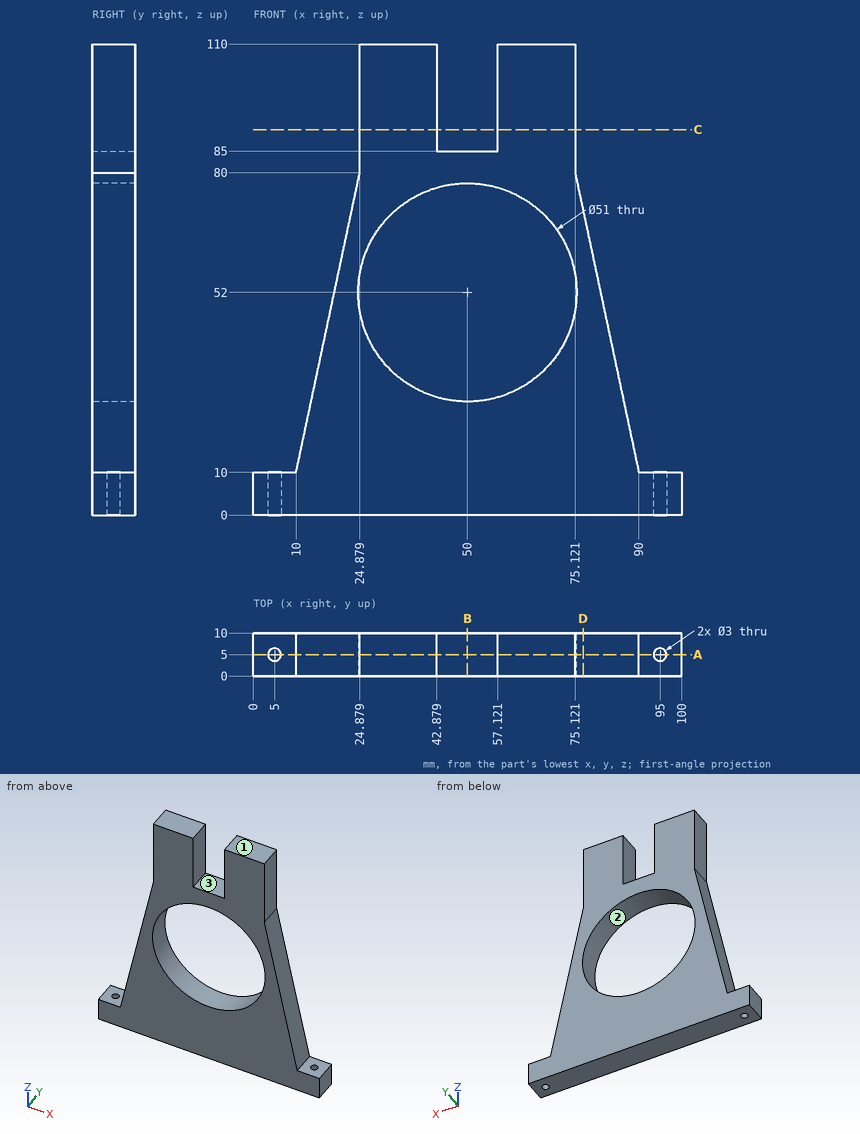
Here's the drawing with two shaded views (mm, measured from the low corner). I have some questions. Give positions to 0.01 mm unless a question says otherwise; leave off trailing zeros. Loops run counter-clockwise (first coordinate to the right, second up) from the corner with the lowest first, then second, coordinate; pieces in that order, holes last. Notation, with made-up numbers: M 81,23.25 L 106,23.25 A33 ccw 106,55.25 Z; hole C 77,-30.75 d2. An arc over 180 degrees is marked long. One line per item, written item: value.
1) Imagine slicing it at C-C on z = 90. Write out the boundary of the cut face in (x, y), and give its area (3 significant figures).
Geometry check:
outline: M 24.88,0 L 42.88,0 L 42.88,10 L 24.88,10 Z; M 57.12,0 L 75.12,0 L 75.12,10 L 57.12,10 Z
area: 360 mm²
2) Please list where these lines run through material, in increasing order: line 1 (Z direction, x = 50, y = 4); line 2 (Y direction, x = 5, z = 5); line 3 (X direction, y = 6.25, z = 6.5).
Geometry check:
line 1: z = 0 to 26.5, 77.5 to 85
line 2: y = 0 to 3.5, 6.5 to 10
line 3: x = 0 to 4.17, 5.83 to 94.17, 95.83 to 100
3) Imagine slicing it at A-A on y = 5. Write out the boundary of the cut face in (x, z), and give its area (3 significant figures).
Geometry check:
outline: M 0,0 L 3.5,0 L 3.5,10 L 0,10 Z; M 6.5,0 L 93.5,0 L 93.5,10 L 90,10 L 75.12,80 L 75.12,110 L 57.12,110 L 57.12,85 L 42.88,85 L 42.88,110 L 24.88,110 L 24.88,80 L 10,10 L 6.5,10 Z; M 96.5,0 L 100,0 L 100,10 L 96.5,10 Z; hole C 50,52 d51
area: 4,610 mm²
4) Imagine slicing it at B-B on x = 50. Write out the boundary of the cut face in (y, z).
Geometry check:
outline: M 0,0 L 10,0 L 10,26.5 L 0,26.5 Z; M 0,77.5 L 10,77.5 L 10,85 L 0,85 Z
5) Imagine slicing it at D-D on x = 77. Write out the boundary of the cut face in (y, z), and give its area (3 significant figures).
Geometry check:
outline: M 0,0 L 10,0 L 10,71.16 L 0,71.16 Z
area: 712 mm²
6) Thinking about a two-plate mould opening in X: for the marked faces 1, 2 and 3, which applies, +X half, -X half, draft (parallel to the pull), parting line (faces both ways), or undercut?
Geometry check:
face 1: draft
face 2: undercut
face 3: undercut
7) I'm going to push flat-ended pins straight in: pin 1 (1.5 mm diameter, centred on y = 2.5, z = 97, fed in from +X); pin 2 (1 mm diameter, centred on x = 52, y = 3, fed in from +Z); pin 3 (6 mm diameter, centred on x = 76.5, y = 5.5, fed in from +Z); pin 4 (1.5 mm diameter, centred on y = 4.5, z = 53, fed in from +X). Where does each tip first touch, or does it pass through?
Geometry check:
pin 1: stops at x = 75.12
pin 2: stops at z = 85
pin 3: stops at z = 110
pin 4: stops at x = 81.02
